For this review, take the finished solid that the model builds, in its own axes (mm). Coordinates: 2 decimals unless noted, no trailing zeros. Write each loop counter-clockwise with the first axis right and the second up, starting at its lowest first coordinate (ties: lowest second). Pieces come first, ordered by that corner, then holes. Notation, with made-up numbers: M 56.5,-8.5 L 99.5,-8.5 A29 cw 99.5,30.5 Z; hole C 8,-26.5 d7. An arc over 180 degrees is marked long. One line per question, with ' | ' between items.
from build123d import *

# Parameters (mm, degrees)
SKETCH1_W            = 200
SKETCH1_H            = 120
BOSS_EXTRUDE1_DEPTH  = 7.9248
SKETCH3_R            = 4.826
CUT_EXTRUDE1_DEPTH   = 153.521481946
LPATTERN1_COUNT      = 3
LPATTERN1_PITCH      = 80
LPATTERN1_COUNT_DIR2 = 2
LPATTERN1_PITCH_DIR2 = 80
SKETCH6_R            = 12.5
CUT_EXTRUDE2_DEPTH   = 153.521481946


with BuildPart() as part:
    # Sketch1 → Boss-Extrude1 (new body)
    with BuildSketch(Plane(origin=(0, 0, 0), x_dir=(1, 0, 0), z_dir=(0, 1, 0))):
        with Locations((40, 0)):
            Rectangle(SKETCH1_W, SKETCH1_H)
    extrude(amount=BOSS_EXTRUDE1_DEPTH)

    # Sketch3 → Cut-Extrude1 (cut, through all)
    with BuildSketch(Plane(origin=(0, 7.9248, 0), x_dir=(1, 0, 0), z_dir=(0, 1, 0))):
        with Locations(Location((-40, 40, 0), (0, 0, 270))):
            Circle(SKETCH3_R)
    cut_extrude1 = extrude(amount=-CUT_EXTRUDE1_DEPTH, mode=Mode.SUBTRACT)

    # LPattern1: Cut-Extrude1 3 × 2
    with Locations(*[(i * LPATTERN1_PITCH, 0, j * LPATTERN1_PITCH_DIR2) for i in range(LPATTERN1_COUNT) for j in range(LPATTERN1_COUNT_DIR2) if (i, j) != (0, 0)]):
        add(cut_extrude1, mode=Mode.SUBTRACT)

    # Sketch6 → Cut-Extrude2 (cut, through all)
    with BuildSketch(Plane(origin=(0, 7.9248, 0), x_dir=(1, 0, 0), z_dir=(0, 1, 0))):
        with Locations(Location((0, 0, 0), (0, 0, 270))):
            Circle(SKETCH6_R)
    extrude(amount=-CUT_EXTRUDE2_DEPTH, mode=Mode.SUBTRACT)


solid = part.part
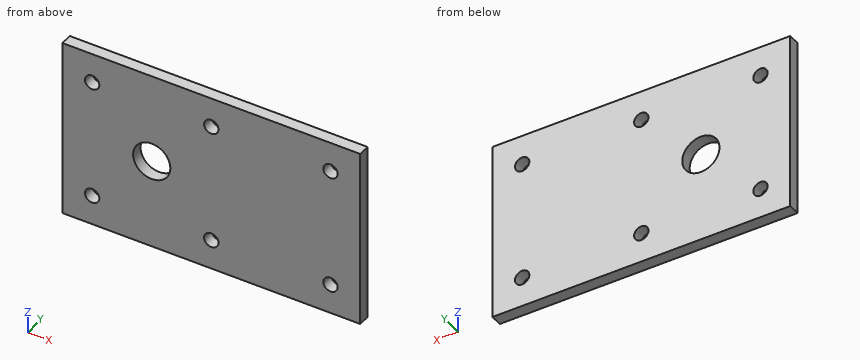
1. Take a section at B-B on y = 5.5. State the section outline as (x, z) points, plus the area to 3 significant figures.
Computed values:
outline: M -60,-60 L 140,-60 L 140,60 L -60,60 Z; hole C -40,-40 d9.65; hole C -40,40 d9.65; hole C 0,0 d25; hole C 40,-40 d9.65; hole C 40,40 d9.65; hole C 120,-40 d9.65; hole C 120,40 d9.65 | area: 23,100 mm2
2. For line 1 along X through (y, z) = (3.5, -40); line 2 along X through (y, z) = (5, 0); line 3 along Z through (x, y) = (37, 4.5), list the stretches that pass through material, from the lowest coordinate up.
Computed values:
line 1: x = -60 to -44.83, -35.17 to 35.17, 44.83 to 115.17, 124.83 to 140 | line 2: x = -60 to -12.5, 12.5 to 140 | line 3: z = -60 to -43.78, -36.22 to 36.22, 43.78 to 60
3. Take a section at D-D on z = -40. State the section outline as (x, y) points.
Computed values:
outline: M -60,0 L -44.83,0 L -44.83,7.92 L -60,7.92 Z; M -35.17,0 L 35.17,0 L 35.17,7.92 L -35.17,7.92 Z; M 44.83,0 L 115.17,0 L 115.17,7.92 L 44.83,7.92 Z; M 124.83,0 L 140,0 L 140,7.92 L 124.83,7.92 Z
4. Take a section at C-C on x = -40. State the section outline as (y, z) points, plus the area to 3 significant figures.
Computed values:
outline: M 0,-60 L 7.92,-60 L 7.92,-44.83 L 0,-44.83 Z; M 0,-35.17 L 7.92,-35.17 L 7.92,35.17 L 0,35.17 Z; M 0,44.83 L 7.92,44.83 L 7.92,60 L 0,60 Z | area: 798 mm2
5. Take a section at A-A on z = 0. State the section outline as (x, y) points, plus the area to 3 significant figures.
Computed values:
outline: M -60,0 L -12.5,0 L -12.5,7.92 L -60,7.92 Z; M 12.5,0 L 140,0 L 140,7.92 L 12.5,7.92 Z | area: 1,390 mm2
